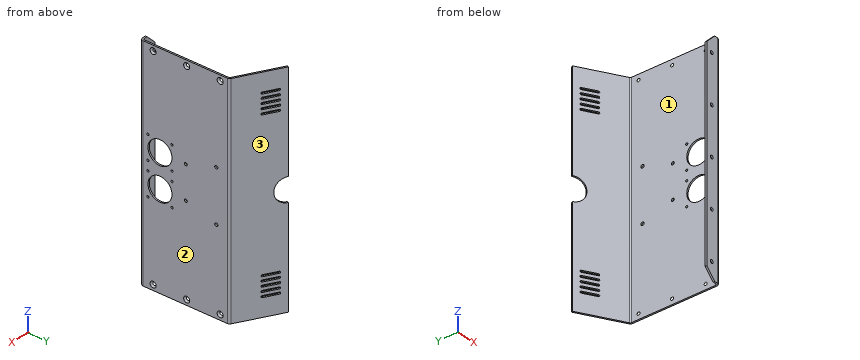
```python
from build123d import *

# Parameters (mm, degrees)
BASE_FLANGE1_DEPTH = 235
SKETCH6_R          = 3.5
CUT_EXTRUDE1_DEPTH = 10
CHAMFER1_SIZE      = 20
SKETCH8_R          = 3
CUT_EXTRUDE3_DEPTH = 3.26
SKETCH11_R         = 2.286
SKETCH11_R_2       = 25
CUT_EXTRUDE5_DEPTH = 3.26
SKETCH12_R         = 3
CUT_EXTRUDE6_DEPTH = 10
CUT_EXTRUDE7_DEPTH = 10
CUT_EXTRUDE8_DEPTH = 10
CHAMFER2_SIZE      = 3.3
SKETCH15_R         = 3.375
CUT_EXTRUDE9_DEPTH = 10


# Sheet-metal steps are written as plain solids
with BuildPart() as part:
    # Sketch1 → Base-Flange1 (new, symmetric)
    with BuildSketch(Plane.XY):
        with BuildLine():
            Line((-30, 0), (-3.048, 0))
            ThreePointArc((-3.048, 0), (-0.892738531, 0.892738531), (0, 3.048))
            Line((0, 3.048), (0, 178.24023638))
            ThreePointArc((0, 178.24023638), (-0.408354569, 179.76423638), (-1.524, 180.87988181))
            Line((-1.524, 180.87988181), (-86.602540378, 230))
            Line((-86.602540378, 230), (-84.972540378, 232.823242816))
            Line((-84.972540378, 232.823242816), (0.106, 183.703124627))
            ThreePointArc((0.106, 183.703124627), (2.414888247, 181.39423638), (3.26, 178.24023638))
            Line((3.26, 178.24023638), (3.26, 3.048))
            ThreePointArc((3.26, 3.048), (1.412429576, -1.412429576), (-3.048, -3.26))
            Line((-3.048, -3.26), (-30, -3.26))
            Line((-30, -3.26), (-30, 0))
        make_face()
    extrude(amount=BASE_FLANGE1_DEPTH, both=True)

    # Sketch6 → Cut-Extrude1 (cut)
    with BuildSketch(Plane(origin=(0, 0, 0), x_dir=(1, 0, 0), z_dir=(0, 1, 0))):
        with Locations(Location((-17.387, 0.59516, 0), (0, 0, 270))):
            Circle(SKETCH6_R)
        with Locations(Location((-17.387, -199.40484, 0), (0, 0, 270))):
            Circle(SKETCH6_R)
        with Locations(Location((-17.387, -99.40484, 0), (0, 0, 270))):
            Circle(SKETCH6_R)
        with Locations(Location((-17.387, 200.59516, 0), (0, 0, 270))):
            Circle(SKETCH6_R)
        with Locations(Location((-17.387, 100.59516, 0), (0, 0, 270))):
            Circle(SKETCH6_R)
    extrude(amount=-CUT_EXTRUDE1_DEPTH, mode=Mode.SUBTRACT)

    # Chamfer1
    chamfer1_edges = [part.edges().sort_by_distance(p)[0] for p in [
        (-30, -1.63, -235),
        (-30, -1.63, 235),
    ]]
    chamfer(chamfer1_edges, length=CHAMFER1_SIZE)

    # Sketch8 → Cut-Extrude3 (cut)
    with BuildSketch(Plane(origin=(3.26, 0, 0), x_dir=(0, 0, -1), z_dir=(1, 0, 0))):
        with Locations((-223.61916, 163.426)):
            Circle(SKETCH8_R)
        with Locations((-223.61916, 93.576)):
            Circle(SKETCH8_R)
        with Locations((-223.61916, 23.726)):
            Circle(SKETCH8_R)
        with Locations(Location((223.61916, 23.726, 0), (0, 0, 180))):
            Circle(SKETCH8_R)
        with Locations(Location((223.61916, 93.576, 0), (0, 0, 180))):
            Circle(SKETCH8_R)
        with Locations(Location((223.61916, 163.426, 0), (0, 0, 180))):
            Circle(SKETCH8_R)
    extrude(amount=-CUT_EXTRUDE3_DEPTH, mode=Mode.SUBTRACT)

    # Sketch11 → Cut-Extrude5 (cut)
    with BuildSketch(Plane(origin=(3.26, 0, 0), x_dir=(0, 0, -1), z_dir=(1, 0, 0))):
        with Locations(Location((-60, 63.048, 0), (0, 0, 90))):
            Circle(SKETCH11_R)
        with Locations(Location((-10, 63.048, 0), (0, 0, 90))):
            Circle(SKETCH11_R)
        with Locations(Location((-10, 13.048, 0), (0, 0, 90))):
            Circle(SKETCH11_R)
        with Locations(Location((-60, 13.048, 0), (0, 0, 90))):
            Circle(SKETCH11_R)
        with Locations(Location((-35, 38.048, 0), (0, 0, 90))):
            Circle(SKETCH11_R_2)
        with Locations(Location((35, 38.048, 0), (0, 0, 180))):
            Circle(SKETCH11_R_2)
        with Locations(Location((60, 13.048, 0), (0, 0, 180))):
            Circle(SKETCH11_R)
        with Locations(Location((10, 13.048, 0), (0, 0, 180))):
            Circle(SKETCH11_R)
        with Locations(Location((10, 63.048, 0), (0, 0, 180))):
            Circle(SKETCH11_R)
        with Locations(Location((60, 63.048, 0), (0, 0, 180))):
            Circle(SKETCH11_R)
    extrude(amount=-CUT_EXTRUDE5_DEPTH, mode=Mode.SUBTRACT)

    # Sketch12 → Cut-Extrude6 (cut)
    with BuildSketch(Plane.ZY):
        with Locations((35, 91.949)):
            Circle(SKETCH12_R)
        with Locations((-35, 91.949)):
            Circle(SKETCH12_R)
    extrude(amount=-CUT_EXTRUDE6_DEPTH, mode=Mode.SUBTRACT)

    # Sketch13 → Cut-Extrude7 (cut)
    with BuildSketch(Plane(origin=(79.572286341, 137.823242816, 0), x_dir=(0.8660254037844399, -0.4999999999999977, 0), z_dir=(0.4999999999999977, 0.8660254037844399, 0))):
        with BuildLine():
            Line((-175, 197), (-145, 197))
            ThreePointArc((-145, 197), (-143, 195), (-145, 193))
            Line((-145, 193), (-175, 193))
            ThreePointArc((-175, 193), (-177, 195), (-175, 197))
        make_face()
        with BuildLine():
            Line((-175, 187), (-145, 187))
            ThreePointArc((-145, 187), (-143, 185), (-145, 183))
            Line((-145, 183), (-175, 183))
            ThreePointArc((-175, 183), (-177, 185), (-175, 187))
        make_face()
        with BuildLine():
            Line((-175, 177), (-145, 177))
            ThreePointArc((-145, 177), (-143, 175), (-145, 173))
            Line((-145, 173), (-175, 173))
            ThreePointArc((-175, 173), (-177, 175), (-175, 177))
        make_face()
        with BuildLine():
            Line((-175, 167), (-145, 167))
            ThreePointArc((-145, 167), (-143, 165), (-145, 163))
            Line((-145, 163), (-175, 163))
            ThreePointArc((-175, 163), (-177, 165), (-175, 167))
        make_face()
        with BuildLine():
            Line((-175, 157), (-145, 157))
            ThreePointArc((-145, 157), (-143, 155), (-145, 153))
            Line((-145, 153), (-175, 153))
            ThreePointArc((-175, 153), (-177, 155), (-175, 157))
        make_face()
        with BuildLine():
            Line((-175, -197), (-145, -197))
            ThreePointArc((-145, -197), (-143, -195), (-145, -193))
            Line((-145, -193), (-175, -193))
            ThreePointArc((-175, -193), (-177, -195), (-175, -197))
        make_face()
        with BuildLine():
            Line((-175, -187), (-145, -187))
            ThreePointArc((-145, -187), (-143, -185), (-145, -183))
            Line((-145, -183), (-175, -183))
            ThreePointArc((-175, -183), (-177, -185), (-175, -187))
        make_face()
        with BuildLine():
            Line((-175, -177), (-145, -177))
            ThreePointArc((-145, -177), (-143, -175), (-145, -173))
            Line((-145, -173), (-175, -173))
            ThreePointArc((-175, -173), (-177, -175), (-175, -177))
        make_face()
        with BuildLine():
            Line((-175, -167), (-145, -167))
            ThreePointArc((-145, -167), (-143, -165), (-145, -163))
            Line((-145, -163), (-175, -163))
            ThreePointArc((-175, -163), (-177, -165), (-175, -167))
        make_face()
        with BuildLine():
            Line((-175, -157), (-145, -157))
            ThreePointArc((-145, -157), (-143, -155), (-145, -153))
            Line((-145, -153), (-175, -153))
            ThreePointArc((-175, -153), (-177, -155), (-175, -157))
        make_face()
    extrude(amount=-CUT_EXTRUDE7_DEPTH, mode=Mode.SUBTRACT)

    # Sketch14 → Cut-Extrude8 (cut)
    with BuildSketch(Plane(origin=(79.572286341, 137.823242816, 0), x_dir=(0.8660254037844399, -0.4999999999999977, 0), z_dir=(0.4999999999999977, 0.8660254037844399, 0))):
        with BuildLine():
            Line((-190, 25), (-190, -25))
            ThreePointArc((-190, -25), (-165, 0), (-190, 25))
        make_face()
    extrude(amount=-CUT_EXTRUDE8_DEPTH, mode=Mode.SUBTRACT)

    # Chamfer2
    # the kernel refuses this chamfer: 3.3 mm, written as the material it takes off along each edge
    with BuildSketch(Plane(origin=(3.26, 163.426, -223.61916), x_dir=(0, 0, 1), z_dir=(0, 1, 0))) as chamfer2_piece_1:
        Polygon((3 + CHAMFER2_SIZE, 0), (3, -CHAMFER2_SIZE), (3, 0), align=None)
    revolve(axis=Axis((3.26, 163.426, -223.61916), (1, 0, 0)), mode=Mode.SUBTRACT)
    with BuildSketch(Plane(origin=(3.26, 93.576, -223.61916), x_dir=(0, 0, 1), z_dir=(0, 1, 0))) as chamfer2_piece_2:
        Polygon((3 + CHAMFER2_SIZE, 0), (3, -CHAMFER2_SIZE), (3, 0), align=None)
    revolve(axis=Axis((3.26, 93.576, -223.61916), (1, 0, 0)), mode=Mode.SUBTRACT)
    with BuildSketch(Plane(origin=(3.26, 23.726, -223.61916), x_dir=(0, 0, 1), z_dir=(0, 1, 0))) as chamfer2_piece_3:
        Polygon((3 + CHAMFER2_SIZE, 0), (3, -CHAMFER2_SIZE), (3, 0), align=None)
    revolve(axis=Axis((3.26, 23.726, -223.61916), (1, 0, 0)), mode=Mode.SUBTRACT)
    with BuildSketch(Plane(origin=(3.26, 23.726, 223.61916), x_dir=(0, 0, -1), z_dir=(0, -1, 0))) as chamfer2_piece_4:
        Polygon((3 + CHAMFER2_SIZE, 0), (3, -CHAMFER2_SIZE), (3, 0), align=None)
    revolve(axis=Axis((3.26, 23.726, 223.61916), (1, 0, 0)), mode=Mode.SUBTRACT)
    with BuildSketch(Plane(origin=(3.26, 93.576, 223.61916), x_dir=(0, 0, -1), z_dir=(0, -1, 0))) as chamfer2_piece_5:
        Polygon((3 + CHAMFER2_SIZE, 0), (3, -CHAMFER2_SIZE), (3, 0), align=None)
    revolve(axis=Axis((3.26, 93.576, 223.61916), (1, 0, 0)), mode=Mode.SUBTRACT)
    with BuildSketch(Plane(origin=(3.26, 163.426, 223.61916), x_dir=(0, 0, -1), z_dir=(0, -1, 0))) as chamfer2_piece_6:
        Polygon((3 + CHAMFER2_SIZE, 0), (3, -CHAMFER2_SIZE), (3, 0), align=None)
    revolve(axis=Axis((3.26, 163.426, 223.61916), (1, 0, 0)), mode=Mode.SUBTRACT)

    # Sketch15 → Cut-Extrude9 (cut)
    with BuildSketch(Plane(origin=(3.26, 0, 0), x_dir=(0, 0, -1), z_dir=(1, 0, 0))):
        with Locations((-55, 155.24023638)):
            Circle(SKETCH15_R)
        with Locations((55, 155.24023638)):
            Circle(SKETCH15_R)
    extrude(amount=-CUT_EXTRUDE9_DEPTH, mode=Mode.SUBTRACT)


solid = part.part
```
For this review, take the finished solid that the model builds, in its own axes (mm). Face numbers are marked on the shaded views. Round coordinates to 2 decimals unless told otherwise and drop trailing zeros. Order: outer loops, then holes, each group sorted by start corner. A loop starts at its lowest first (then second) coordinate and runs counter-clockwise, first axis right, second up.
Q1. Mouldability with a two-part tool opening along Y and no side actions: class the marked faces 1, 2 and 3 as pulls with the +Y half, pulls with the -Y half, needs draft (parallel to the pull), parting line crosses it, or undercut.
Findings below:
face 1: undercut
face 2: needs draft
face 3: pulls with the +Y half
Q2. Wall thickness on line 1 (X direction, y = 40.5, z = -82.5); line 2 (Y direction, x = -11, z = -39.5); line 3 (Y direction, x = -46.5, z = -205): over which ranges is each line inside the solid? List them lowest first.
Findings below:
line 1: x = 0 to 3.26
line 2: y = -3.26 to 0, 186.35 to 190.12
line 3: y = 206.85 to 210.61
Q3. Insertion check: P1, Ø4, axis at y = 13.048, z = 60, coming from the -X side; P2, Ø8, axis at x = -42.5, z = 120.5, coming from the -Y side; P3, Ø4, axis at x = -35, z = -27.5, coming from the +Y side; P4, Ø2, axis at y = 57.5, z = -58, coming from the -X side. Each pin has a flat end and moves straight along its axis. Give the tip position at first contact, or say it passes through.
Findings below:
P1: passes through
P2: stops at y = 202.23
P3: stops at y = 205.13
P4: stops at x = 0
Q4. We need section A-A, the plane z = 45. Give the boundary of the cut face in (x, y), plus the area to 3 significant figures.
Findings below:
outline: (-86.6, 230) - (-1.52, 180.88) arc R3.05 cw to (0, 178.24) - (0, 60.96) - (3.26, 60.96) - (3.26, 178.24) arc R6.31 ccw to (0.11, 183.7) - (-84.97, 232.82) - close; (-30, -3.26) - (-3.05, -3.26) arc R6.31 ccw to (3.26, 3.05) - (3.26, 15.14) - (0, 15.14) - (0, 3.05) arc R3.05 cw to (-3.05, 0) - (-30, 0) - close
area: 870 mm2
Q5. We need section B-B, the plane z = -80. Give the boundary of the cut face in (x, y).
Findings below:
outline: (-86.6, 230) - (-1.52, 180.88) arc R3.05 cw to (0, 178.24) - (0, 3.05) arc R3.05 cw to (-3.05, 0) - (-30, 0) - (-30, -3.26) - (-3.05, -3.26) arc R6.31 ccw to (3.26, 3.05) - (3.26, 178.24) arc R6.31 ccw to (0.11, 183.7) - (-84.97, 232.82) - close
Q6. We need section C-C, the plane y = 127.5. Give the boundary of the cut face in (x, z).
Findings below:
outline: (0, -235) - (3.26, -235) - (3.26, 235) - (0, 235) - close
